CAD build for the part. Positions are in the model's coordinates, mm. Face numbers are marked on the shaded views. Round coordinates to 2 decimals unless told otherwise and drop trailing zeros. Write each loop counter-clockwise with the first axis right and the second up, starting at its lowest first coordinate (ties: lowest second). Pieces come first, ordered by that corner, then holes. Notation, with made-up numbers: (14.25, 86.25) - (66.25, 86.25) arc R24 cw to (66.25, 103.25) - close; hole circle Ø8 at (68.25, 29.5). An arc over 180 degrees is marked (long way). Use one line per item in the form item = value. Start each with the question number.
Item 1: Band-saw the part on A-A, the plane y = 0. List the corners of the cut face in (x, z), and give its area (3 significant figures).
Item 2: Pin check, flat tip, straight feed: pin 1 (8 mm diameter, centred on x = -46.5, y = 39, fed in from -Z). Stop position of the tip, or through.
Item 3: Pull direction X, two halves, no side cores. Call the marked faces 1 and 2: +X half, -X half, draft (parallel to the pull), parting line (faces both ways), or undercut.
Item 4: Band-saw the part on C-C, the plane z = 4.15. List the corners of the cut face in (x, y).
Item 5: Drill centre lines: L1, parallel to X at y = 20.5, z = 0.3; L2, parallel to Y at x = -17, z = 1.85; L3, parallel to Z at x = -35.5, y = 46. Where is each one in solid material? Low to high.
Item 6: Band-saw the part on D-D, the plane y = 33.5. List the corners of the cut face in (x, z), and give its area (3 significant figures).
Item 7: Band-saw the part on B-B, the plane x = 32.5. List the corners of the cut face in (y, z).
from build123d import *

# Parameters (mm, degrees)
F1_DEPTH = 5.08
F2_T     = -2.54
F4_D     = 20


with BuildPart() as f1:
    # F0 (on Top) → F1 (new body)
    with BuildSketch(Plane.XY):
        with BuildLine():
            Line((-74.373494, -50.733282), (79.453494, -50.733282))
            ThreePointArc((79.453494, -50.733282), (80.35152, -50.361307), (80.723494, -49.463282))
            Line((80.723494, -49.463282), (80.723494, 44.383282))
            ThreePointArc((80.723494, 44.383282), (78.863622, 48.87341), (74.373494, 50.733282))
            Line((74.373494, 50.733282), (-74.373494, 50.733282))
            ThreePointArc((-74.373494, 50.733282), (-78.863622, 48.87341), (-80.723494, 44.383282))
            Line((-80.723494, 44.383282), (-80.723494, -44.383282))
            ThreePointArc((-80.723494, -44.383282), (-78.863622, -48.87341), (-74.373494, -50.733282))
        make_face()
    extrude(amount=F1_DEPTH)

    # F2
    f2_openings = [f1.faces().sort_by_distance(p)[0] for p in [
        (0.040257, -0.025024, 0),
    ]]
    offset(amount=F2_T, openings=f2_openings)

    # F4 (through all)
    with Locations(Plane(origin=(0, 0, 0), x_dir=(1, 0, 0), z_dir=(0, 0, -1))):
        with Locations((-38.540371, 0)):
            Hole(F4_D / 2)


solid = f1.part
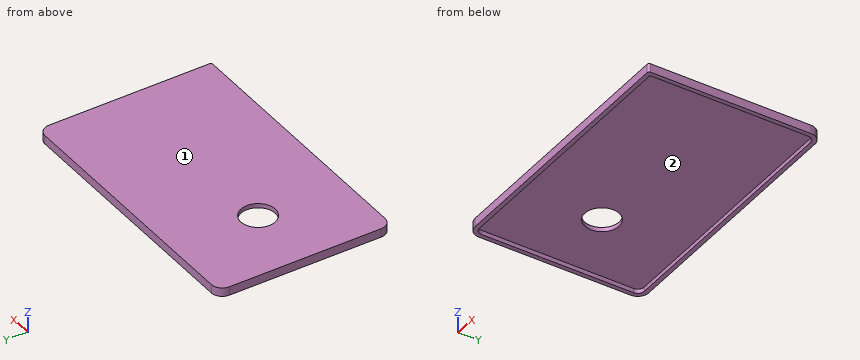
Determined:
q1.outline = (-80.72, 0) - (-78.18, 0) - (-78.18, 2.54) - (-48.54, 2.54) - (-48.54, 5.08) - (-80.72, 5.08) - close; (-28.54, 2.54) - (78.18, 2.54) - (78.18, 0) - (80.72, 0) - (80.72, 5.08) - (-28.54, 5.08) - close
q1.area = 372 mm²
q2.pin_1 = 2.54
q3.face_1 = draft
q3.face_2 = undercut
q4.outline = (-80.72, -44.38) arc R6.35 ccw to (-74.37, -50.73) - (79.45, -50.73) arc R1.27 ccw to (80.72, -49.46) - (80.72, 44.38) arc R6.35 ccw to (74.37, 50.73) - (-74.37, 50.73) arc R6.35 ccw to (-80.72, 44.38) - close; hole circle Ø20 at (-38.54, 0)
q5.L1 = -80.72 to -78.18, 78.18 to 80.72
q5.L2 = -50.73 to -48.19, 48.19 to 50.73
q5.L3 = 2.54 to 5.08
q6.outline = (-80.72, 0) - (-78.18, 0) - (-78.18, 2.54) - (78.18, 2.54) - (78.18, 0) - (80.72, 0) - (80.72, 5.08) - (-80.72, 5.08) - close
q6.area = 423 mm²
q7.outline = (-50.73, 0) - (-48.19, 0) - (-48.19, 2.54) - (48.19, 2.54) - (48.19, 0) - (50.73, 0) - (50.73, 5.08) - (-50.73, 5.08) - close
